```python
from build123d import *

# Parameters (mm, degrees)
SKETCH1_R               = 12.7
EXTRUDE1_DEPTH          = 51.816
SKETCH2_R               = 9.525
EXTRUDE2_DEPTH          = 7
SKETCH3_R               = 5.5626
EXTRUDE3_DEPTH          = 20.178
SKETCH4_W               = 4
SKETCH4_H               = 12
CUT_EXTRUDE1_DEPTH      = 10
SKETCH5_R               = 1.5
CUT_EXTRUDE2_DEPTH      = 10
CUT_EXTRUDE2_DEPTH_BACK = 10


with BuildPart() as part:
    # Sketch1 → Extrude1 (new body)
    with BuildSketch(Plane.XY):
        Circle(SKETCH1_R)
    extrude(amount=EXTRUDE1_DEPTH)

    # Sketch2 → Extrude2 (add)
    with BuildSketch(Plane.XY.offset(51.816)):
        Circle(SKETCH2_R)
    extrude(amount=EXTRUDE2_DEPTH)

    # Sketch3 → Extrude3 (add)
    with BuildSketch(Plane.XY.offset(58.816)):
        Circle(SKETCH3_R)
    extrude(amount=EXTRUDE3_DEPTH)

    # Sketch4 → Cut-Extrude1 (cut)
    with BuildSketch(Plane.XY.offset(78.994)):
        Rectangle(SKETCH4_W, SKETCH4_H)
    extrude(amount=-CUT_EXTRUDE1_DEPTH, mode=Mode.SUBTRACT)

    # Sketch5 → Cut-Extrude2 (cut, two sides)
    with BuildSketch(Plane.ZY.offset(-2)) as cut_extrude2_sk:
        with Locations((73.994, 0.000618341)):
            Circle(SKETCH5_R)
    extrude(amount=CUT_EXTRUDE2_DEPTH, mode=Mode.SUBTRACT)
    extrude(cut_extrude2_sk.sketch, amount=-CUT_EXTRUDE2_DEPTH_BACK, mode=Mode.SUBTRACT)


solid = part.part
```
Build history of the part. All positions in model axes, mm. A direction names the side the tool comes from. Round coordinates to 2 decimals unless told otherwise and drop trailing zeros. Write each loop counter-clockwise with the first axis right and the second up, starting at its lowest first coordinate (ties: lowest second). Pieces come first, ordered by that corner, then holes. Notation, with made-up numbers: (30.5, -25) - (50.5, -25) arc R30 ccw to (50.5, 12) - close; hole circle Ø5 at (55, 16). An arc over 180 degrees is marked (long way). Answer as CSV lines item,"result".
Q1. Cut at C-C (y = 8). Write the cut outline in (x, z).
Report:
outline,"(-9.86, 0) - (9.86, 0) - (9.86, 51.82) - (5.17, 51.82) - (5.17, 58.82) - (-5.17, 58.82) - (-5.17, 51.82) - (-9.86, 51.82) - close"
Q2. Cut at A-A (x = -3). Write the cut outline in (y, z), and give its area (3 significant figures).
Report:
outline,"(-12.34, 0) - (12.34, 0) - (12.34, 51.82) - (9.04, 51.82) - (9.04, 58.82) - (4.68, 58.82) - (4.68, 78.99) - (-4.68, 78.99) - (-4.68, 58.82) - (-9.04, 58.82) - (-9.04, 51.82) - (-12.34, 51.82) - close; hole circle Ø3 at (0, 73.99)"
area,"1,590 mm^2"
Q3. Cut at D-D (x = 7). Write the cut outline in (y, z).
Report:
outline,"(-10.6, 0) - (10.6, 0) - (10.6, 51.82) - (6.46, 51.82) - (6.46, 58.82) - (-6.46, 58.82) - (-6.46, 51.82) - (-10.6, 51.82) - close"
Q4. Drill centre lines: probe 1 along Z at (x, y) = (7.25, -0.75); probe 2 along Z at (x, y) = (-11.25, 1.5); probe 3 along Y at (x, z) = (0.5, 19.5). Where is each one in solid material? Low to high. Write a range as [from, to].
Report:
probe 1,"z = [0, 58.82]"
probe 2,"z = [0, 51.82]"
probe 3,"y = [-12.69, 12.69]"
Q5. Pull direction Z, two halves, no side cores. Call faces 4 (the cylindrical face through (3.756, 0.067, 72.495)), 5 (the cylindrical face through (-3.756, 0.067, 72.495)), 6 (the flat face through (0, 0, 0)), 7 (the flat face through (2, -1.2, 75.2)): +Z half, -Z half, draft (parallel to the pull), parting line (faces both ways), or undercut.
Report:
face 4,"undercut"
face 5,"undercut"
face 6,"-Z half"
face 7,"draft"
Q6. Drop flat-ended pins along their axis: pin 1 (3.5 mm diameter, centred on y = 0, z = 73.99, fed in from -X); pin 2 (1.2 mm diameter, centred on x = 0, y = 1, fed in from +Z); pin 3 (1.5 mm diameter, centred on x = 0.5, z = 53.5, fed in from -Y) (3 decimals). Give the stop position or say it passes through.
Report:
pin 1,"stops at x = -5.56"
pin 2,"stops at z = 68.99"
pin 3,"stops at y = -9.525"
Q7. Cut at B-B (z = 63). Write the cut outline in (x, y), and give its area (3 significant figures).
Report:
outline,"circle Ø11.13 at (0, 0)"
area,"97.2 mm^2"
Q8. Tool access for faces 1 (the flat face through (0, 0, 68.994)), 2 (the flat face through (4.1, -4.1, 58.816)), 3 (the flat face through (-3, 0, 78.994)): list every direction of +Z, -Z, +X, -X, +Y, -Y with a clear straight run to the whole face (end or side of a thin tool).
Report:
face 1,"+Z, +Y, -Y"
face 2,"+Z"
face 3,"+Z, +X, -X, +Y, -Y"
